```python
from build123d import *

# Parameters (mm, degrees)
EXTRUDE_2_DEPTH     = 192
SKETCH_5_R          = 60
CUT_EXTRUDE_2_DEPTH = 167
SKETCH_6_R          = 65
CUT_EXTRUDE_3_DEPTH = 167
EXTRUDE_3_DEPTH     = 81
SKETCH_8_W          = 31.710893006
SKETCH_8_H          = 3.805307161
EXTRUDE_4_DEPTH     = 7
SKETCH_9_W          = 9.753754566
SKETCH_9_H          = 1.960413463
CUT_EXTRUDE_4_DEPTH = 3
FILLET_1_R          = 3
EXTRUDE_5_DEPTH     = 3


with BuildPart() as part:
    # 草图4 → 凸台-拉伸2 (new body)
    with BuildSketch(Plane.XY):
        with BuildLine():
            Line((-63.444815749, -57.709462621), (-34.077926376, -57.709462621))
            ThreePointArc((-34.077926376, -57.709462621), (0, 67.020050299), (34.077926376, -57.709462621))
            Line((34.077926376, -57.709462621), (69.007018872, -57.709462621))
            Line((69.007018872, -57.709462621), (73.554721348, -69.931413026))
            Line((73.554721348, -69.931413026), (-69.697906654, -69.931413026))
            Line((-69.697906654, -69.931413026), (-63.444815749, -57.709462621))
        make_face()
    extrude(amount=EXTRUDE_2_DEPTH)

    # 草图5 → 切除-拉伸2 (cut)
    with BuildSketch(Plane(origin=(0, 0, 0), x_dir=(-1, 0, 0), z_dir=(0, 0, -1))):
        Circle(SKETCH_5_R)
    extrude(amount=-CUT_EXTRUDE_2_DEPTH, mode=Mode.SUBTRACT)

    # 草图6 → 切除-拉伸3 (cut)
    with BuildSketch(Plane(origin=(0, 0, 0), x_dir=(-1, 0, 0), z_dir=(0, 0, -1))):
        Circle(SKETCH_6_R)
    extrude(amount=-CUT_EXTRUDE_3_DEPTH, mode=Mode.SUBTRACT)

    # 草图7 → 凸台-拉伸3 (add)
    with BuildSketch(Plane(origin=(0, 0, 0), x_dir=(-1, 0, 0), z_dir=(0, 0, -1))):
        with BuildLine():
            Line((-47.897732915, -41.016239679), (-50.424875633, -41.016239679))
            ThreePointArc((-50.424875633, -41.016239679), (0, -65), (50.424875633, -41.016239679))
            Line((50.424875633, -41.016239679), (47.897732915, -41.016239679))
            ThreePointArc((47.897732915, -41.016239679), (0, -63.059691846), (-47.897732915, -41.016239679))
        make_face()
    extrude(amount=-EXTRUDE_3_DEPTH)

    # 草图8 → 凸台-拉伸4 (add)
    with BuildSketch(Plane(origin=(0, 0, 0), x_dir=(-1, 0, 0), z_dir=(0, 0, -1))):
        with Locations((0.108672156, -65.494898904)):
            Rectangle(SKETCH_8_W, SKETCH_8_H)
    extrude(amount=EXTRUDE_4_DEPTH)

    # 草图9 → 切除-拉伸4 (cut)
    with BuildSketch(Plane(origin=(0, 0, -7), x_dir=(-1, 0, 0), z_dir=(0, 0, -1))):
        with Locations((0, -65.811506795)):
            Rectangle(SKETCH_9_W, SKETCH_9_H)
    extrude(amount=-CUT_EXTRUDE_4_DEPTH, mode=Mode.SUBTRACT)

    # 圆角1
    # the kernel refuses this fillet: 3 mm, written as the material it takes off along each edge
    with BuildSketch(Plane(origin=(-4.876877283, -66.791713526, -7), x_dir=(-1, 0, 0), z_dir=(0, 1, 0)), Plane(origin=(4.876877283, -64.831300063, -7), x_dir=(1, 0, 0), z_dir=(0, -1, 0))) as fillet_1_piece_1:
        with BuildLine():
            CenterArc((FILLET_1_R, FILLET_1_R), FILLET_1_R, 180, 90)
            Line((0, FILLET_1_R), (-FILLET_1_R * 0.02, FILLET_1_R))
            Line((-FILLET_1_R * 0.02, FILLET_1_R), (-FILLET_1_R * 0.02, -FILLET_1_R * 0.02))
            Line((-FILLET_1_R * 0.02, -FILLET_1_R * 0.02), (FILLET_1_R, -FILLET_1_R * 0.02))
            Line((FILLET_1_R, -FILLET_1_R * 0.02), (FILLET_1_R, 0))
        make_face()
    extrude(amount=1.960413463, mode=Mode.SUBTRACT)
    with BuildSketch(Plane(origin=(-4.876877283, -64.831300063, -7), x_dir=(0, 1, 0), z_dir=(1, 0, 0))) as fillet_1_piece_2:
        with BuildLine():
            CenterArc((FILLET_1_R, FILLET_1_R), FILLET_1_R, 180, 90)
            Line((0, FILLET_1_R), (-FILLET_1_R * 0.02, FILLET_1_R))
            Line((-FILLET_1_R * 0.02, FILLET_1_R), (-FILLET_1_R * 0.02, -FILLET_1_R * 0.02))
            Line((-FILLET_1_R * 0.02, -FILLET_1_R * 0.02), (FILLET_1_R, -FILLET_1_R * 0.02))
            Line((FILLET_1_R, -FILLET_1_R * 0.02), (FILLET_1_R, 0))
        make_face()
    extrude(amount=9.753754565, mode=Mode.SUBTRACT)
    with BuildSketch(Plane(origin=(-12.376877283, -64.831300063, -7), x_dir=(0, 1, 0), z_dir=(1, 0, 0))) as fillet_1_piece_3a_section:
        with BuildLine():
            CenterArc((FILLET_1_R, FILLET_1_R), FILLET_1_R, 180, 90)
            Line((0, FILLET_1_R), (-FILLET_1_R * 0.02, FILLET_1_R))
            Line((-FILLET_1_R * 0.02, FILLET_1_R), (-FILLET_1_R * 0.02, -FILLET_1_R * 0.02))
            Line((-FILLET_1_R * 0.02, -FILLET_1_R * 0.02), (FILLET_1_R, -FILLET_1_R * 0.02))
            Line((FILLET_1_R, -FILLET_1_R * 0.02), (FILLET_1_R, 0))
        make_face()
    fillet_1_piece_3a = extrude(amount=17.253754565, mode=Mode.PRIVATE)
    fillet_1_piece_3a = split(fillet_1_piece_3a, bisect_by=Plane(origin=(-4.876877283, -64.15211472, -6.320814657), z_dir=(-1, 0, 0)), keep=Keep.TOP, mode=Mode.PRIVATE)
    with BuildSketch(Plane(origin=(-4.876877283, -66.791713526, -7), x_dir=(-1, 0, 0), z_dir=(0, 1, 0))) as fillet_1_piece_3b_section:
        with BuildLine():
            CenterArc((FILLET_1_R, FILLET_1_R), FILLET_1_R, 180, 90)
            Line((0, FILLET_1_R), (-FILLET_1_R * 0.02, FILLET_1_R))
            Line((-FILLET_1_R * 0.02, FILLET_1_R), (-FILLET_1_R * 0.02, -FILLET_1_R * 0.02))
            Line((-FILLET_1_R * 0.02, -FILLET_1_R * 0.02), (FILLET_1_R, -FILLET_1_R * 0.02))
            Line((FILLET_1_R, -FILLET_1_R * 0.02), (FILLET_1_R, 0))
        make_face()
    fillet_1_piece_3b = extrude(amount=9.460413463, mode=Mode.PRIVATE)
    fillet_1_piece_3b = split(fillet_1_piece_3b, bisect_by=Plane(origin=(-5.556062626, -64.831300063, -6.320814657), z_dir=(0, 1, 0)), keep=Keep.TOP, mode=Mode.PRIVATE)
    fillet_1_piece_3 = fillet_1_piece_3a & fillet_1_piece_3b
    add(fillet_1_piece_3, mode=Mode.SUBTRACT)
    with BuildSketch(Plane(origin=(4.876877283, -57.331300063, -7), x_dir=(1, 0, 0), z_dir=(0, -1, 0))) as fillet_1_piece_4a_section:
        with BuildLine():
            CenterArc((FILLET_1_R, FILLET_1_R), FILLET_1_R, 180, 90)
            Line((0, FILLET_1_R), (-FILLET_1_R * 0.02, FILLET_1_R))
            Line((-FILLET_1_R * 0.02, FILLET_1_R), (-FILLET_1_R * 0.02, -FILLET_1_R * 0.02))
            Line((-FILLET_1_R * 0.02, -FILLET_1_R * 0.02), (FILLET_1_R, -FILLET_1_R * 0.02))
            Line((FILLET_1_R, -FILLET_1_R * 0.02), (FILLET_1_R, 0))
        make_face()
    fillet_1_piece_4a = extrude(amount=9.460413463, mode=Mode.PRIVATE)
    fillet_1_piece_4a = split(fillet_1_piece_4a, bisect_by=Plane(origin=(5.556062626, -64.831300063, -6.320814657), z_dir=(0, 1, 0)), keep=Keep.TOP, mode=Mode.PRIVATE)
    with BuildSketch(Plane(origin=(-4.876877283, -64.831300063, -7), x_dir=(0, 1, 0), z_dir=(1, 0, 0))) as fillet_1_piece_4b_section:
        with BuildLine():
            CenterArc((FILLET_1_R, FILLET_1_R), FILLET_1_R, 180, 90)
            Line((0, FILLET_1_R), (-FILLET_1_R * 0.02, FILLET_1_R))
            Line((-FILLET_1_R * 0.02, FILLET_1_R), (-FILLET_1_R * 0.02, -FILLET_1_R * 0.02))
            Line((-FILLET_1_R * 0.02, -FILLET_1_R * 0.02), (FILLET_1_R, -FILLET_1_R * 0.02))
            Line((FILLET_1_R, -FILLET_1_R * 0.02), (FILLET_1_R, 0))
        make_face()
    fillet_1_piece_4b = extrude(amount=17.253754565, mode=Mode.PRIVATE)
    fillet_1_piece_4b = split(fillet_1_piece_4b, bisect_by=Plane(origin=(4.876877283, -64.15211472, -6.320814657), z_dir=(1, 0, 0)), keep=Keep.TOP, mode=Mode.PRIVATE)
    fillet_1_piece_4 = fillet_1_piece_4a & fillet_1_piece_4b
    add(fillet_1_piece_4, mode=Mode.SUBTRACT)

    # 草图10 → 凸台-拉伸5 (add)
    with BuildSketch(Plane.XY.offset(81)):
        with BuildLine():
            Line((-49.354840822, -43.055078484), (49.354840822, -43.055078484))
            ThreePointArc((49.354840822, -43.055078484), (0, -65.495344078), (-49.354840822, -43.055078484))
        make_face()
    extrude(amount=EXTRUDE_5_DEPTH)


solid = part.part
```
Input: part model. Units: mm. Frame: model coordinates. A direction names the side the tool comes from. Give positions to 0.01 mm unless a question says otherwise; leave off trailing zeros. Order: outer loops, then holes, each group sorted by start corner. A loop starts at its lowest first (then second) coordinate and runs counter-clockwise, first axis right, second up. Notation, with made-up numbers: (44.25, 39.25) -> (65.25, 39.25) arc R18 cw to (65.25, 54.25) -> close; hole circle Ø3 at (-28, 42.5). An arc over 180 degrees is marked (long way). Write each question's results on one line, items separated by ' | '. Start each with the question number.
Item 1: Cut plane C-C on x = 0. Return the cut outline in (y, z), then the cut area to 3 significant figures.
Item 2: Cut plane D-D on z = 71.5. Return the cut outline in (x, y).
Item 3: Cut plane A-A on z = 93.5. Return the cut outline in (x, y).
Item 4: Line query: line 1 (Y direction, x = 0, z = 93); line 2 (X direction, y = 0, z = 117); line 3 (Y direction, x = -46, z = 92.5). Output: solid intervals per line, ascending.
Item 5: Contact query for flat-ended pins moving along their axis: P1, Ø14.5, axis at x = -53, z = 95.5, coming from the +Y side; P2, Ø2, axis at y = 39, z = 116, coming from the +X side; P3, Ø1.1, axis at y = -65, z = -3.5, coming from the +X side; P4, Ø7.5, axis at x = -5, z = -3.5, coming from the -Y side. Output: stop coordinate, or through.
Item 6: Mould query, pull axis Y, two halves, no side actions, for faces 1 (the flat face through (13, -62, 0)), 2 (the cylindrical face through (-0.762, -63.055, 39.933)), 3 (the flat face through (3, -69.931, 95)). Classes: pulls with the +Y half, pulls with the -Y half, needs draft (parallel to the pull), parting line crosses it, or undercut.
Item 7: Cut plane B-B on y = 0. Return the cut outline in (x, z), then the cut area to 3 significant figures.
Item 8: Set-up query: faces 4 (the flat face through (-66.615, -63.906, 94.656)), 5 (the flat face through (0, -67.398, -3)), 6 (the flat face through (1, -51, 81)). Return all of +Z, -Z, +X, -X, +Y, -Y with unobstructed straight access to the full face (end or side cutting, diameter ignored); none if empty.
Established:
1) outline: (-69.93, 0) -> (-67.4, 0) -> (-67.4, -7) -> (-66.79, -7) -> (-66.79, -4) -> (-64.83, -4) arc R3 ccw to (-63.59, -6.43) -> (-63.59, 0) -> (-63.06, 0) -> (-63.06, 81) -> (-43.06, 81) -> (-43.06, 84) -> (-65, 84) -> (-65, 167) -> (65, 167) -> (65, 0) -> (67.02, 0) -> (67.02, 192) -> (-69.93, 192) -> close | area: 4,830 mm^2
2) outline: (-69.7, -69.93) -> (73.55, -69.93) -> (69.01, -57.71) -> (34.08, -57.71) arc R67.02 ccw (long way) to (-34.08, -57.71) -> (-63.44, -57.71) -> close; hole (-50.42, -41.02) -> (-47.9, -41.02) arc R63.06 ccw to (47.9, -41.02) -> (50.42, -41.02) arc R65 ccw (long way) to start
3) outline: (-69.7, -69.93) -> (73.55, -69.93) -> (69.01, -57.71) -> (34.08, -57.71) arc R67.02 ccw (long way) to (-34.08, -57.71) -> (-63.44, -57.71) -> close; hole circle Ø130 at (0, 0)
4) line 1: -69.93 to -65, 65 to 67.02 | line 2: -67.02 to -65, 65 to 67.02 | line 3: -69.93 to -57.71, -48.74 to -45.92, 45.92 to 48.74
5) P1: y = 48.98 | P2: x = 55.21 | P3: x = 15.75 | P4: y = -69.93
6) face 1: needs draft | face 2: undercut | face 3: pulls with the -Y half
7) outline: (-67.02, 0) -> (-65, 0) -> (-65, 167) -> (65, 167) -> (65, 0) -> (67.02, 0) -> (67.02, 192) -> (-67.02, 192) -> close | area: 4,030 mm^2
8) face 4: +Z, -Z, -X | face 5: -Z, +X, -X, -Y | face 6: -Z
